from build123d import *

# Parameters (mm, degrees)
SKETCH1_W          = 25.4
SKETCH1_H          = 2.413
CHAMFER1_SIZE      = 0.5953125
CUT_EXTRUDE2_DEPTH = 1.79578
SKETCH6_R          = 1.833087105
CUT_EXTRUDE3_DEPTH = 1.79578
CUT_EXTRUDE3_TAPER = 45


with BuildPart() as part:
    # Sketch1 → Revolve1 (revolve)
    with BuildSketch(Plane(origin=(0, 0, 0), x_dir=(0, 0, -1), z_dir=(1, 0, 0))):
        with Locations((15.2654, 1.2065)):
            Rectangle(SKETCH1_W, SKETCH1_H)
    revolve(axis=Axis((0, 0, -27.9654), (0, 0, 1)))

    # Chamfer1
    chamfer1_edges = [part.edges().sort_by_distance(p)[0] for p in [
        (0, -2.413, -27.9654),
    ]]
    chamfer(chamfer1_edges, length=CHAMFER1_SIZE)

    # Sketch7 → Revolve2 (revolve)
    with BuildSketch(Plane(origin=(0, 0, 0), x_dir=(0, 0, -1), z_dir=(1, 0, 0)), mode=Mode.PRIVATE) as revolve2_sk:
        with BuildLine():
            Line((2.18059, 4.5847), (2.5654, 4.5847))
            Line((2.5654, 4.5847), (2.5654, 0))
            Line((2.5654, 0), (0, 0))
            Line((0, 0), (0, 2.413))
            ThreePointArc((0, 2.413), (0.925030326, 3.664791196), (2.18059, 4.5847))
        make_face()
    revolve(revolve2_sk.sketch.rotate(Axis((0, 0, 0), (0, 0, -1)), 180), axis=Axis((0, 0, 0), (0, 0, -1)))

    # Sketch5 → Cut-Extrude2 (cut)
    with BuildSketch(Plane.XY):
        Polygon((1.5875, -0.916543552), (1.5875, 0.916543552), (0, 1.833087105), (-1.5875, 0.916543552), (-1.5875, -0.916543552), (0, -1.833087105), align=None)
    extrude(amount=-CUT_EXTRUDE2_DEPTH, mode=Mode.SUBTRACT)

    # Sketch6 → Cut-Extrude3 (cut)
    with BuildSketch(Plane.XY):
        Circle(SKETCH6_R)
    extrude(amount=-CUT_EXTRUDE3_DEPTH, taper=CUT_EXTRUDE3_TAPER, mode=Mode.SUBTRACT)


solid = part.part
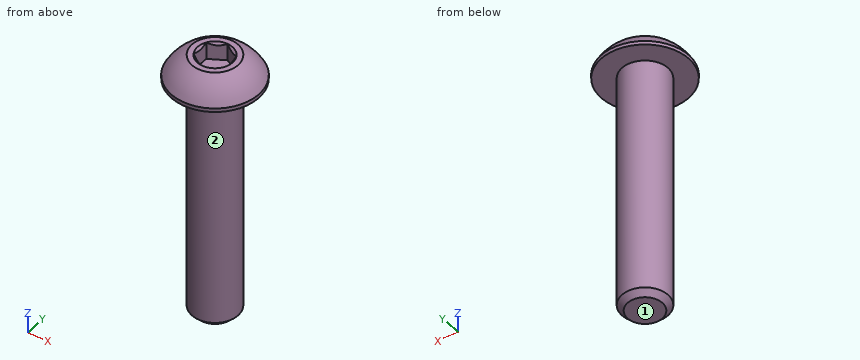
Model file for the job. Use its own axes, mm. Face numbers are marked on the shaded views. A direction names the side the tool comes from. Give positions to 0.01 mm unless a question says otherwise; leave off trailing zeros. Order: outer loops, then holes, each group sorted by start corner. A loop starts at its lowest first (then second) coordinate and runs counter-clockwise, first axis right, second up. Notation, with made-up numbers: M 14,51 L 29,51 A23 ccw 29,66 Z; hole C 44,-3.5 d1. An arc over 180 degrees is marked long. Write item = value, one per line.
Q1. Cut at C-C, the plane x = -3.75. List the corners of the cut face in (y, z).
Derived:
outline = M -2.64,-2.57 L 2.64,-2.57 L 2.64,-2.18 A3.56 ccw -2.64,-2.18 Z
Q2. Drill centre lines: line 1 (Z direction, x = 0, y = 1.25); line 2 (Z direction, x = 0.75, y = -1.75); line 3 (Y direction, x = 2.5, z = -2). Where is each one in solid material? Low to high. Write a range as [from, to].
Derived:
line_1 = [-27.97, -1.8]
line_2 = [-27.88, 0]
line_3 = [-3.72, 3.72]
Q3. Cut at A-A, the plane z = -19.5. List the corners of the cut face in (x, y), then the cut area to 3 significant figures.
Derived:
outline = C 0,0 d4.83
area = 18.3 mm2
Q4. Cut at B-B, the plane x = 4. List the corners of the cut face in (y, z), then the cut area to 3 significant figures.
Derived:
outline = M -2.24,-2.57 L 2.24,-2.57 L 2.24,-2.18 A3.28 ccw -2.24,-2.18 Z
area = 4.45 mm2
Q5. Flat gauge pins, fed straight in: pin 1 (1.5 mm diameter, centred on x = -1.5, z = -11.5, fed in from +Y); pin 2 (0.5 mm diameter, centred on y = 0, z = -0.5, fed in from +X); pin 3 (5 mm diameter, centred on x = -3, z = -20, fed in from -Y). Where does each tip first touch, or does it go through?
Derived:
pin_1 = 2.29
pin_2 = 3.48
pin_3 = -2.36
Q6. Tool access for the marked faces 1 and 2: list every direction of +Z, -Z, +X, -X, +Y, -Y with a clear straight run to the whole face (end or side of a thin tool).
Derived:
face_1 = -Z, +X, -X, +Y, -Y
face_2 = -Z
